Verification items for the finished model (mm, model axes). A direction names the side the tool comes from. Round coordinates to 2 decimals unless told otherwise and drop trailing zeros. Loops run counter-clockwise (first coordinate to the right, second up) from the corner with the lowest first, then second, coordinate; pieces in that order, holes last. Notation, with made-up numbers: (89, -8.75) -> (125, -8.75) arc R25 ccw to (125, 30.25) -> close; hole circle Ø8 at (68.5, -33.75). An arc over 180 degrees is marked (long way). Use a Markdown table: item, result. Add a question column.
Autodesk Inventor part; units mm, degrees
ref_plane "YZ Plane" through (0, 0, 0) normal (1, 0, 0) x (0, 1, 0)
ref_plane "XY Plane" through (0, 0, 0) normal (0, 0, 1) x (1, 0, 0)
ref_plane "Work Plane1" through (-71.4709, -34.2956, -57.6282) normal (0, 0, -1) x (-1, 0, 0)
sketch "Sketch1" plane through (-71.4709, -34.2956, -57.6282) normal (0, 0, -1) x (-1, 0, 0)
  circle A0 centre (0, 0) radius 17.93
  point P0 (-71.4709, 34.2956)
extrude "Extrusion1" add sketch "Sketch1" along normal blind 0.8
sketch "Sketch2" plane through (-71.4709, -34.2956, -57.6282) normal (0, 0, 1) x (1, 0, 0)
  circle A0 centre (0, 0) radius 12.175 construction
  circle A1 centre (12.175, 0) radius 1.415
  circle A2 centre (-12.175, 0) radius 1.415
  point P0 (71.4709, 34.2956)
  dimension "d2" = 24.35
  dimension "d3" = 2.83
  dimension "d4" = 2.83
extrude "Extrusion2" cut sketch "Sketch2" against normal blind 0.8
sketch "Sketch3" plane through (-71.4709, -34.2956, -57.6282) normal (0, 0, 1) x (1, 0, 0)
  circle A0 centre (0, 0) radius 6.5
  point P0 (71.4709, 34.2956)
  dimension "d7" = 13
extrude "Extrusion3" add sketch "Sketch3" along normal blind 4.5
fillet "Fillet1" radius 0.508 1 edges at (-77.9709, -34.2956, -53.1282)
sketch "Sketch4" plane through (-71.4709, -34.2956, -53.1282) normal (0, 0, 1) x (1, 0, 0)
  circle A0 centre (0, 0) radius 1.6
  point P0 (71.4709, 34.2956)
  dimension "d11" = 3.2
extrude "Extrusion4" cut sketch "Sketch4" against normal blind 19.2875
properties part number "capot_inf" material "Iron, Cast"
1) Access from +Z, -Z, +X, -X, +Y, -Y to the whole of each face (thin tool, end or side, straight path). Record for faces 1 (the face through (-70, -36, -53.128)), 2 (the face through (-79, -34, -57.628)).
2) Thickness scan on line 1 (Y direction, x = -71.5, z = -56.2); line 2 (Z direction, x = -59, y = -38); line 3 (X direction, y = -29.5, z = -56). Record the ranges inside material, lowest first.
3) Sectioned sample at D-D on y = -33.5. State how many separate pieces and enclosed holes the cut face has, then the cut area to 3 significant figures.
4) Release check for a two-part mould opening along X. For faces 3 (the face through (-71, -38, -58.428)), 4 (the face through (-76.6, -30.3, -55.7)), 5 (the face through (-82.34, -34.84, -58.02)), 6 (the face through (-60.71, -34.23, -58.02)) record: released by +X, released by -X, zero draft, split by the parting line, or undercut.
5) Sectioned sample at C-C on x = -81.5. Enter the section's corners in (y, z), then the cut area to 3 significant figures.
6) Sectioned sample at A-A on y = -47. Enter the section's corners in (x, z).
7) Go/stop test with flat-tipped pins: pin 1 (2.5 mm diameter, centred on x = -59.3, y = -34.3, fed in from -Z); pin 2 (3 mm diameter, centred on y = -36, z = -55.5, fed in from +X); pin 3 (2 mm diameter, centred on x = -69, z = -54, fed in from -Y); pin 4 (3 mm diameter, centred on x = -63, z = -57, fed in from -Y). Record where each tip stops, or that it passes through.
8) Sectioned sample at B-B on z = -55.4. Enter the section's corners in (x, y).
Geometry results:
| question | item | result |
|---|---|---|
| 1 | face 1 | +Z, +X, -X, +Y, -Y |
| 1 | face 2 | +Z |
| 2 | line 1 | -40.8 to -35.9, -32.7 to -27.8 |
| 2 | line 2 | -58.43 to -57.63 |
| 2 | line 3 | -75.86 to -67.08 |
| 3 | separate pieces | 4 |
| 3 | enclosed holes | 0 |
| 3 | area | 68.1 mm^2 |
| 4 | face 3 | zero draft |
| 4 | face 4 | split by the parting line |
| 4 | face 5 | undercut |
| 4 | face 6 | undercut |
| 5 | outline | (-49.16, -58.43) -> (-19.43, -58.43) -> (-19.43, -57.63) -> (-49.16, -57.63) -> close |
| 5 | area | 23.8 mm^2 |
| 6 | outline | (-84.12, -58.43) -> (-58.82, -58.43) -> (-58.82, -57.63) -> (-84.12, -57.63) -> close |
| 7 | pin 1 | through |
| 7 | pin 2 | x = -64.97 |
| 7 | pin 3 | y = -40.63 |
| 7 | pin 4 | y = -50.76 |
| 8 | outline | circle Ø13 at (-71.47, -34.3); hole circle Ø3.2 at (-71.47, -34.3) |
